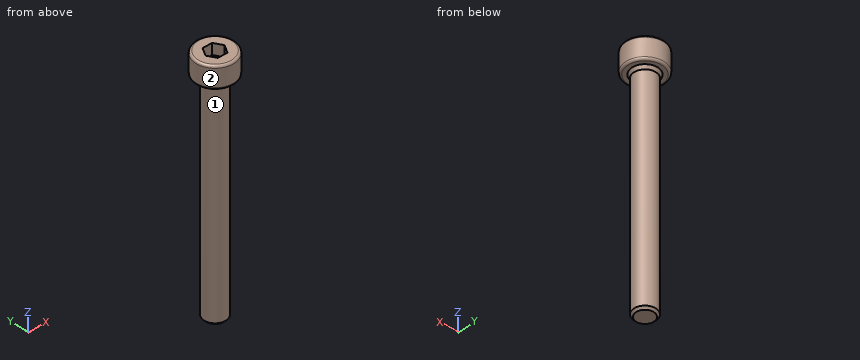
Solid Edge part; units mm, degrees
sketch "Sketch1" plane through (0, 0, 0) normal (0, -1, 0) x (1, 0, 0)
  line L0 (3.5, 4) -> (3.5, 0)
  line L1 (3.5, 0) -> (2.35, 0)
  line L2 (2.35, 0) -> (2, -0.6062)
  line L3 (2, -0.6062) -> (2, -40)
  line L4 (2, -40) -> (0, -40)
  line L5 (1.5, 2) -> (0, 1.834)
  line L6 (1.5, 4) -> (1.5, 2)
  line L7 (3.5, 4) -> (1.5, 4)
revolve "RevolvedProtrusion1" add sketch "Sketch1" angle 360 about axis through (0, 0, -6) along (0, 0, 1)
cosmetic_thread "Thread1"
chamfer "Chamfer_1" distance 0.4 angle 45 1 edges at (-2, 0, -40)
fillet "Round_1" radius 0.4 2 edges at (-3.5, 0, 0) (-3.5, 0, 4)
sketch "Sketch2" plane through (0, 0, 4) normal (0, 0, 1) x (0, 1, 0)
  line L0 (-1.5, 0.866) -> (-1.5, -0.866)
  line L1 (0, -1.7321) -> (-1.5, -0.866)
  line L2 (1.5, -0.866) -> (0, -1.7321)
  line L3 (1.5, 0.866) -> (1.5, -0.866)
  line L4 (0, 1.7321) -> (1.5, 0.866)
  line L5 (-1.5, 0.866) -> (0, 1.7321)
extrude "Cutout1" cut sketch "Sketch2" against normal up to vertex (2 mm away)
properties material "Galvanized steel"
Geometry: final body of the model. Coordinates: model frame, mm. Face numbers are marked on the shaded views. A direction names the side the tool comes from. Coordinates: 2 decimals unless noted, no trailing zeros. Order: outer loops, then holes, each group sorted by start corner. A loop starts at its lowest first (then second) coordinate and runs counter-clockwise, first axis right, second up. Notation, with made-up numbers: (69.5, 39.25) - (83.5, 39.25) arc R19 ccw to (83.5, 51.25) - close; hole circle Ø9 at (-25.75, 3.25). An arc over 180 degrees is marked (long way). Write each question's results on one line, items separated by ' | '.
1) Line query: line 1 (Y direction, x = 0, z = -31); line 2 (X direction, y = 1, z = -9); line 3 (Z direction, x = 2.5, y = -1). Output: solid intervals per line, ascending. Write a range as from..to.
Results list:
line 1: -2..2 | line 2: -1.73..1.73 | line 3: 0..4
2) Set-up query: the marked faces 1 and 2. Return all of +Z, -Z, +X, -X, +Y, -Y with unobstructed straight access to the full face (end or side cutting, diameter ignored); none if empty.
Results list:
face 1: -Z | face 2: +Z, -Z
3) Pin query (flat end, axial travel): pin 1 (0.5 mm diameter, centred on x = -1, y = 0.5, fed in from +Z); pin 2 (1.5 mm diameter, centred on y = 1, z = -27.5, fed in from -X). Return the tip coordinate at first contact, or that it passes through.
Results list:
pin 1: z = 1.99 | pin 2: x = -1.98
4) Section A-A, the plane z = -15. Return loops of the section in (x, y), plus the area to 3 significant figures.
Results list:
outline: circle Ø4 at (0, 0) | area: 12.6 mm^2
